Can you work these out from the model? Positions are in its coordinate system, mm. A direction names the side the tool comes from. Give positions to 0.01 mm unless a question says otherwise; leave off trailing zeros. Loops run counter-clockwise (first coordinate to the right, second up) from the corner with the lowest first, then second, coordinate; pieces in that order, holes last. Notation, with made-up numbers: (-32.5, 36.25) -> (24.5, 36.25) arc R21 cw to (24.5, 58.25) -> close; hole circle Ø3 at (-37.75, 28.5). An arc over 180 degrees is marked (long way). Return JSON: item names as keys, results as strings. Group by question number.
Q1. Suppose I cut it at D-D, the plane z = 8. Please give me the cut outline in (x, y).
Q2. Which directions (+Z, -Z, +X, -X, +Y, -Y) give clear straight access to the entire face, cutting with the end or side of a thin tool? Please do faces 1 (the flat face through (6, 44, 5)), 2 (the flat face through (11, 0, 4)), 3 (the flat face through (1, 32, 4)), 4 (the flat face through (7.1, 34, 8.6)), 5 (the flat face through (16, 32, 4)).
Q3. Will these pins go through, and if not, where does the flat tip stop? pin 1 (0.6 mm diameter, centred on y = 33, z = 2.5, fed in from -X); pin 2 (1.6 mm diameter, centred on y = 33.5, z = 3, fed in from +X); pin 3 (0.8 mm diameter, centred on x = 1, z = 6.5, fed in from +Y).
Q4. Suppose I cut it at B-B, the plane x = 6. Please give me the cut outline in (y, z).
Q5. I need wall thicknesses on line 1 along Y through (x, z) = (15.25, 8.25); line 2 along Z through (x, y) = (5.5, 40.5); line 3 along X through (y, z) = (40, 3.5). Which ranges of each line are inside material? Lowest first, please. Write a range as [from, to].
Q6. Suppose I cut it at C-C, the plane x = 17.75. Please give me the cut outline in (y, z).
Q7. Suppose I cut it at A-A, the plane z = 4.5. Please give me the cut outline in (x, y), and give its area (3 significant figures).
```python
from build123d import *

# Parameters (mm, degrees)
F0_W     = 22
F0_H     = 32
F1_DEPTH = 9
F2_W     = 9
F2_H     = 9
F3_DEPTH = 2
F4_R     = 4
F5_DEPTH = 10


with BuildPart() as f1:
    # F0 (on Top) → F1 (new body)
    with BuildSketch(Plane.XY):
        with Locations((11, 16)):
            Rectangle(F0_W, F0_H)
    extrude(amount=F1_DEPTH)

    # F2 (on face) → F3 (join)
    with BuildSketch(Plane(origin=(0, 32, 0), x_dir=(-1, 0, 0), z_dir=(0, 1, 0))):
        with Locations((-6, 4.5)):
            Rectangle(F2_W, F2_H)
    extrude(amount=F3_DEPTH)

    # F4 (on face) → F5 (join)
    with BuildSketch(Plane(origin=(0, 34, 0), x_dir=(-1, 0, 0), z_dir=(0, 1, 0))):
        with Locations((-6, 4.5)):
            Circle(F4_R)
    extrude(amount=F5_DEPTH)


solid = f1.part
```
Ans:
{
 "1": {"outline": "(0, 0) -> (22, 0) -> (22, 32) -> (10.5, 32) -> (10.5, 34) -> (7.94, 34) -> (7.94, 44) -> (4.06, 44) -> (4.06, 34) -> (1.5, 34) -> (1.5, 32) -> (0, 32) -> close"},
 "2": {"face 1": "+Z, -Z, +X, -X, +Y", "face 2": "+Z, -Z, +X, -X, -Y", "face 3": "+Z, -Z, -X, +Y", "face 4": "+Y", "face 5": "+Z, -Z, +X, +Y"},
 "3": {"pin 1": "stops at x = 1.5", "pin 2": "stops at x = 10.5", "pin 3": "stops at y = 32"},
 "4": {"outline": "(0, 0) -> (34, 0) -> (34, 0.5) -> (44, 0.5) -> (44, 8.5) -> (34, 8.5) -> (34, 9) -> (0, 9) -> close"},
 "5": {"line 1": "y = [0, 32]", "line 2": "z = [0.53, 8.47]", "line 3": "x = [2.13, 9.87]"},
 "6": {"outline": "(0, 0) -> (32, 0) -> (32, 9) -> (0, 9) -> close"},
 "7": {"outline": "(0, 0) -> (22, 0) -> (22, 32) -> (10.5, 32) -> (10.5, 34) -> (10, 34) -> (10, 44) -> (2, 44) -> (2, 34) -> (1.5, 34) -> (1.5, 32) -> (0, 32) -> close", "area": "802 mm^2"}
}
